Part model, mm, in its own coordinate system. Round coordinates to 2 decimals unless told otherwise and drop trailing zeros. Write each loop counter-clockwise with the first axis right and the second up, starting at its lowest first coordinate (ties: lowest second). Pieces come first, ordered by that corner, then holes.
1) Saw through at A-A on z = 15. Write the cut outline in (x, y).
2) Flat gauge pin, fed straight in: pin 1 (8 mm diameter, centred on x = -33.5, y = -22.5, fed in from +Z). Where does the tip first touch, or does it go through?
3) Pull direction X, two halves, no side cores. Call faces 1 (the flat face through (100.622, -22, 12)), 2 (the cylindrical face through (68.715, -25.542, 11.591)), 3 (the cylindrical face through (-29.535, -25.542, 11.591)), 4 (the flat face through (-69.378, -22, 12)): +X half, -X half, draft (parallel to the pull), parting line (faces both ways), or undercut.
4) Drill centre lines: L1, parallel to Y at x = 68, z = 13.5; L2, parallel to Y at x = -31.5, z = 13.75. Where is each one in solid material? Low to high.
5) Saw through at B-B on y = -22.5. Write the cut outline in (x, z), and give its area (3 significant figures).
```python
from build123d import *

# Parameters (mm, degrees)
F0_W     = 170
F0_H     = 10
F1_DEPTH = 45
F3_D     = 10


with BuildPart() as f1:
    # F0 (on Front) → F1 (new body)
    with BuildSketch(Plane.XZ):
        with Locations((15.6219, 11.661158)):
            Rectangle(F0_W, F0_H)
    extrude(amount=F1_DEPTH)

    # F3 (through all)
    with Locations(Plane.XY.offset(16.661158)):
        with Locations((-33.5031, -22.5), (64.7469, -22.5)):
            Hole(F3_D / 2)


solid = f1.part
```
Completed:
1. outline: (-69.38, -45) - (100.62, -45) - (100.62, 0) - (-69.38, 0) - close; hole circle Ø10 at (-33.5, -22.5); hole circle Ø10 at (64.75, -22.5)
2. pin 1: passes through
3. face 1: +X half
3. face 2: undercut
3. face 3: undercut
3. face 4: -X half
4. L1: y = -45 to -26.3, -18.7 to 0
4. L2: y = -45 to -27.08, -17.92 to 0
5. outline: (-69.38, 6.66) - (-38.5, 6.66) - (-38.5, 16.66) - (-69.38, 16.66) - close; (-28.5, 6.66) - (59.75, 6.66) - (59.75, 16.66) - (-28.5, 16.66) - close; (69.75, 6.66) - (100.62, 6.66) - (100.62, 16.66) - (69.75, 16.66) - close
5. area: 1,500 mm2
